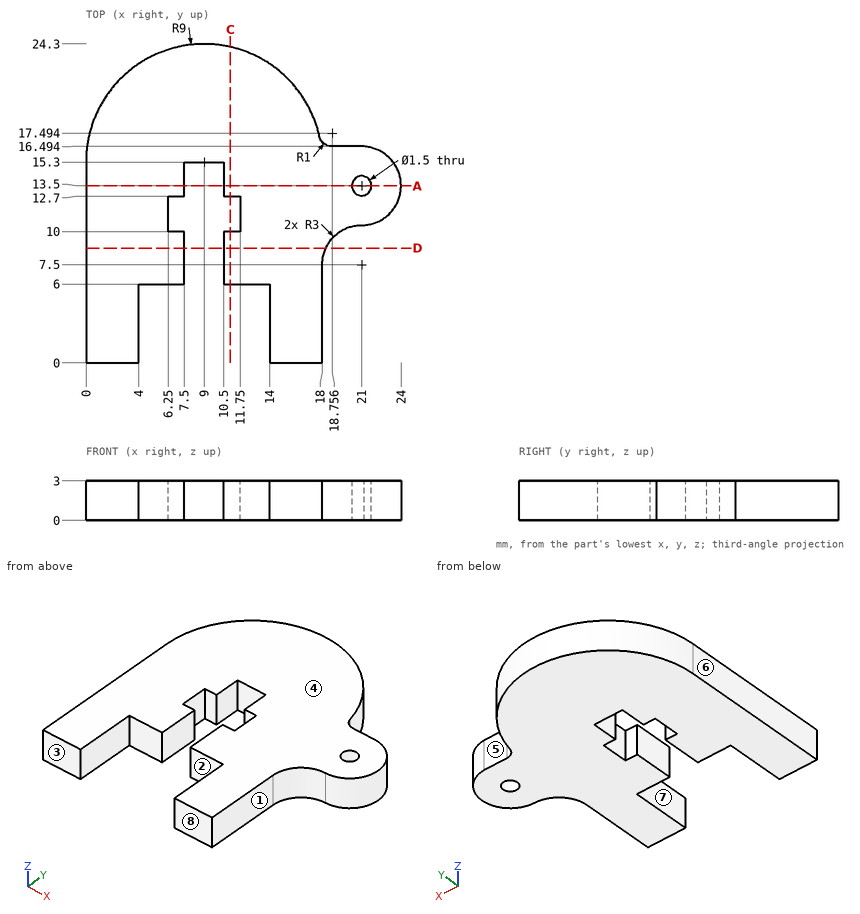
The drawing under review shows one solid part. Ordinate dimensions are in mm from its lowest x, y, z. A direction names the side the tool comes from. Give positions to 0.01 mm unless a question says otherwise; leave off trailing zeros. Order: outer loops, then holes, each group sorted by start corner. A loop starts at its lowest first (then second) coordinate and runs counter-clockwise, first axis right, second up. Notation, with made-up numbers: M -26.75,-28 L 4.25,-28 A26 ccw 4.25,-12 Z; hole C 9,26.25 d5. An arc over 180 degrees is marked long. Answer in a Markdown table with one row per item. Add a question column.
1. Add section C-C on x = 11. State the section outline as (y, z) points (1 decimal).
2. Machinability: for the marked faces 1, 2, 3, 4 and 5, which of the approach directions +Z, -Z, +X, -X, +Y, -Y give a long, thin tool a straight path to every point of the face, cutting with its end or side? Answer none if there is none.
3. For pin 1 Ø1.5 at (x, z) = (9, 2.5) entering from -Y; pin 2 Ø0.6 at (x, z) = (11, 1.5) entering from -Y; pin 3 Ø1.3 at (y, z) = (11.5, 1.5) entering from +X; pin 4 Ø2 at (x, y) = (5, 11) entering from -Z, all flat-tipped, find the tip position at first contact; note any pin that passes through.
4. Add section D-D on y = 8.75. State the section outline as (x, z) points.
5. Mouldability with a two-part tool opening along X and no side actions: class the marked faces 6, 7 and 8 as released by +X, released by -X, zero draft, split by the parting line, or undercut.
6. To check wall thickness, follow line 1 along X through (y, z) = (7.5, 1.75); line 2 along X through (y, z) = (12.25, 1); line 3 along Y through (x, z) = (9.25, 0.5). State the ranges of each line that lie inside material, in increasing order.
7. Add section A-A on y = 13.5. State the section outline as (x, z) points, plus the area to 3 significant figures.
The answers:
| question | item | result |
|---|---|---|
| 1 | outline | M 6,0 L 10,0 L 10,3 L 6,3 Z; M 12.7,0 L 24.1,0 L 24.1,3 L 12.7,3 Z |
| 2 | face 1 | +Z, -Z, +X, -Y |
| 2 | face 2 | +Z, -Z, -Y |
| 2 | face 3 | +Z, -Z, +X, -X, -Y |
| 2 | face 4 | +Z, +X, -X, +Y, -Y |
| 2 | face 5 | +Z, -Z, +X, +Y |
| 3 | pin 1 | y = 15.3 |
| 3 | pin 2 | y = 6 |
| 3 | pin 3 | x = 23.68 |
| 3 | pin 4 | z = 0 |
| 4 | outline | M 0,0 L 7.5,0 L 7.5,3 L 0,3 Z; M 10.5,0 L 18.27,0 L 18.27,3 L 10.5,3 Z |
| 5 | face 6 | released by -X |
| 5 | face 7 | undercut |
| 5 | face 8 | zero draft |
| 6 | line 1 | 0 to 7.5, 10.5 to 18 |
| 6 | line 2 | 0 to 6.25, 11.75 to 23.73 |
| 6 | line 3 | 15.3 to 24.3 |
| 7 | outline | M 0,0 L 7.5,0 L 7.5,3 L 0,3 Z; M 10.5,0 L 20.25,0 L 20.25,3 L 10.5,3 Z; M 21.75,0 L 24,0 L 24,3 L 21.75,3 Z |
| 7 | area | 58.5 mm2 |
